from build123d import *

# Parameters (mm, degrees)
SKETCH_1_W          = 400
SKETCH_1_H          = 329
EXTRUDE_2_DEPTH     = 25
SKETCH_2_W          = 400
SKETCH_2_H          = 9
EXTRUDE_3_DEPTH     = 9
SKETCH_3_W          = 81
SKETCH_3_H          = 27
EXTRUDE_4_DEPTH     = 400
SKETCH_4_W          = 67.25
SKETCH_4_H          = 5
CUT_EXTRUDE_1_DEPTH = 5
CUT_EXTRUDE_2_DEPTH = 400
CUT_EXTRUDE_3_DEPTH = 400
SKETCH_8_R          = 4.5
CUT_EXTRUDE_4_DEPTH = 400


with BuildPart() as part:
    # 草图1 → 凸台-拉伸2 (new body)
    with BuildSketch(Plane(origin=(0, 0, 0), x_dir=(1, 0, 0), z_dir=(0, 1, 0))):
        with Locations((200, 164.5)):
            Rectangle(SKETCH_1_W, SKETCH_1_H)
    extrude(amount=EXTRUDE_2_DEPTH)

    # 草图2 → 凸台-拉伸3 (add)
    with BuildSketch(Plane(origin=(0, 25, 0), x_dir=(1, 0, 0), z_dir=(0, 1, 0))):
        with Locations((200, 324.5)):
            Rectangle(SKETCH_2_W, SKETCH_2_H)
        with Locations((200, 4.5)):
            Rectangle(SKETCH_2_W, SKETCH_2_H)
    extrude(amount=EXTRUDE_3_DEPTH)

    # 草图3 → 凸台-拉伸4 (add)
    with BuildSketch(Plane(origin=(400, 0, 0), x_dir=(0, 0, -1), z_dir=(1, 0, 0))):
        with Locations((205, 38.5)):
            Rectangle(SKETCH_3_W, SKETCH_3_H)
        with Locations((124, 38.5)):
            Rectangle(SKETCH_3_W, SKETCH_3_H)
    extrude(amount=-EXTRUDE_4_DEPTH)

    # 草图4 → 切除-拉伸1 (cut)
    with BuildSketch(Plane.XZ):
        Polygon((200, -5), (200, 0), (133, 0), (133, -329), (267.25, -329), (267.25, -5), align=None)
        with Locations((233.625, -2.5)):
            Rectangle(SKETCH_4_W, SKETCH_4_H)
    extrude(amount=-CUT_EXTRUDE_1_DEPTH, mode=Mode.SUBTRACT)

    # 草图5 → 切除-拉伸2 (cut)
    with BuildSketch(Plane.XY):
        Polygon((133, 5), (133, 8), (118.7, 8), (118.7, 0), (133, 0), align=None)
    extrude(amount=-CUT_EXTRUDE_2_DEPTH, mode=Mode.SUBTRACT)

    # 草图6 → 切除-拉伸3 (cut)
    with BuildSketch(Plane.XY):
        Polygon((118.7, 8), (116.556406461, 0), (118.7, 0), align=None)
    extrude(amount=-CUT_EXTRUDE_3_DEPTH, mode=Mode.SUBTRACT)

    # 草图8 → 切除-拉伸4 (cut)
    with BuildSketch(Plane.XZ):
        with Locations(Location((372.5, -312.4, 0), (0, 0, 270))):
            Circle(SKETCH_8_R)
        with Locations(Location((327.5, -312.4, 0), (0, 0, 270))):
            Circle(SKETCH_8_R)
        with Locations(Location((372.5, -255.4, 0), (0, 0, 270))):
            Circle(SKETCH_8_R)
        with Locations(Location((327.5, -255.4, 0), (0, 0, 270))):
            Circle(SKETCH_8_R)
        with Locations(Location((372.5, -78.5, 0), (0, 0, 270))):
            Circle(SKETCH_8_R)
        with Locations(Location((327.5, -78.5, 0), (0, 0, 270))):
            Circle(SKETCH_8_R)
        with Locations(Location((372.5, -21.5, 0), (0, 0, 270))):
            Circle(SKETCH_8_R)
        with Locations(Location((327.5, -21.5, 0), (0, 0, 270))):
            Circle(SKETCH_8_R)
        with Locations(Location((27.5, -21.5, 0), (0, 0, 270))):
            Circle(SKETCH_8_R)
        with Locations(Location((72.5, -21.5, 0), (0, 0, 270))):
            Circle(SKETCH_8_R)
        with Locations(Location((72.5, -78.5, 0), (0, 0, 270))):
            Circle(SKETCH_8_R)
        with Locations(Location((27.5, -78.5, 0), (0, 0, 270))):
            Circle(SKETCH_8_R)
        with Locations(Location((72.5, -312.4, 0), (0, 0, 270))):
            Circle(SKETCH_8_R)
        with Locations(Location((27.5, -312.4, 0), (0, 0, 270))):
            Circle(SKETCH_8_R)
        with Locations(Location((27.5, -255.4, 0), (0, 0, 270))):
            Circle(SKETCH_8_R)
        with Locations(Location((72.5, -255.4, 0), (0, 0, 270))):
            Circle(SKETCH_8_R)
    extrude(amount=-CUT_EXTRUDE_4_DEPTH, mode=Mode.SUBTRACT)


solid = part.part
Source: CAD feature listing. Evaluate the final solid. Frame: model axes, mm. A direction names the side the tool comes from. Round coordinates to 2 decimals unless told otherwise and drop trailing zeros. Loops run counter-clockwise (first coordinate to the right, second up) from the corner with the lowest first, then second, coordinate; pieces in that order, holes last. Notation, with made-up numbers: (30, 36) - (74, 36) arc R29 ccw to (74, 74) - close; hole circle Ø11 at (-32.75, -18.5). An arc over 180 degrees is marked (long way). Write item = value, one per line. Start each with the question number.
(1) Section query B-B, the plane z = -312.4. Output: boundary loops of the cut face in (x, y), plus the area to 3 significant figures.
(2) Section query A-A, the plane x = 327.5. Output: boundary loops of the cut face in (y, z), plus the area to 3 significant figures.
(3) Section query D-D, the plane z = -175.5. Output: boundary loops of the cut face in (x, y), plus the area to 3 significant figures.
(4) Ray query, line 1 along X through (y, z) = (17.5, -21.5); line 2 along Z through (x, y) = (71, 31); line 3 along Z through (x, y) = (327.5, 11). Return the intervals inside material, ascending. Write a range as from..to.
(5) Pin query (flat end, axial travel): pin 1 (7 mm diameter, centred on x = 281.5, z = -6, fed in from +Y); pin 2 (4.5 mm diameter, centred on x = 231, y = 28, fed in from +Z); pin 3 (11.5 mm diameter, centred on x = 72.5, z = -312.4, fed in from +Y); pin 4 (6 mm diameter, centred on x = 240, z = -246.5, fed in from -Y). Return the tip coordinate at first contact, or that it passes through.
(6) Section query C-C, the plane x = 212.5. Output: boundary loops of the cut face in (y, z).
(7) Set-up query: faces 1 (the face through (197, 34, -325)), 2 (the face through (117.643, 4.056, -162.197)), 3 (the face through (76.96, 12.32, -20.91)), 4 (the face through (197, 25, -47)), 5 (the face through (333, 0, -167)). Return all of +Z, -Z, +X, -X, +Y, -Y with unobstructed straight access to the full face (end or side cutting, diameter ignored); none if empty.
(8) Pull-direction query (X, two-part tool) for faces 6 (the face through (197, 25, -283)), 7 (the face through (0, 20, -162)), 8 (the face through (76.96, 12.32, -77.91)); classes: +X half, -X half, draft (parallel to the pull), parting line (faces both ways), or undercut.
Conclusion:
q1.outline = (0, 0) - (23, 0) - (23, 25) - (0, 25) - close; (32, 0) - (68, 0) - (68, 25) - (32, 25) - close; (77, 0) - (116.56, 0) - (118.7, 8) - (133, 8) - (133, 5) - (267.25, 5) - (267.25, 0) - (323, 0) - (323, 25) - (77, 25) - close; (332, 0) - (368, 0) - (368, 25) - (332, 25) - close; (377, 0) - (400, 0) - (400, 25) - (377, 25) - close
q1.area = 8,310 mm2
q2.outline = (0, -329) - (34, -329) - (34, -320) - (25, -320) - (25, -316.9) - (0, -316.9) - close; (0, -307.9) - (25, -307.9) - (25, -259.9) - (0, -259.9) - close; (0, -250.9) - (25, -250.9) - (25, -245.5) - (52, -245.5) - (52, -83.5) - (25, -83.5) - (25, -83) - (0, -83) - close; (0, -74) - (25, -74) - (25, -26) - (0, -26) - close; (0, -17) - (25, -17) - (25, -9) - (34, -9) - (34, 0) - (0, 0) - close
q2.area = 11,900 mm2
q3.outline = (0, 0) - (116.56, 0) - (118.7, 8) - (133, 8) - (133, 5) - (267.25, 5) - (267.25, 0) - (400, 0) - (400, 52) - (0, 52) - close
q3.area = 20,000 mm2
q4.line_1 = 0..23, 32..68, 77..323, 332..368, 377..400
q4.line_2 = -329..-320, -245.5..-83.5, -9..0
q4.line_3 = -329..-316.9, -307.9..-259.9, -250.9..-83, -74..-26, -17..0
q5.pin_1 = 34
q5.pin_2 = 0
q5.pin_3 = 25
q5.pin_4 = 5
q6.outline = (5, -329) - (34, -329) - (34, -320) - (25, -320) - (25, -245.5) - (52, -245.5) - (52, -83.5) - (25, -83.5) - (25, -9) - (34, -9) - (34, 0) - (5, 0) - close
q7.face_1 = -Z, +X, -X, +Y
q7.face_2 = +Z, -Z, -Y
q7.face_3 = +Y, -Y
q7.face_4 = +X, -X, +Y
q7.face_5 = +Z, -Z, +X, -X, -Y
q8.face_6 = draft
q8.face_7 = -X half
q8.face_8 = undercut
